Read the model definition and answer for the solid it produces. Units are mm, in the model's axes. Coordinates: 2 decimals unless noted, no trailing zeros. Order: outer loops, then holes, each group sorted by start corner. A loop starts at its lowest first (then second) coordinate and runs counter-clockwise, first axis right, second up. Notation, with made-up numbers: (58, 85) -> (110, 85) arc R4 ccw to (110, 90) -> close; hole circle Ø11 at (-10, -35). An arc over 180 degrees is marked (long way). Answer in a Markdown table with one row per item.
from build123d import *

# Parameters (mm, degrees)
SKETCH1_W           = 428.625
SKETCH1_H           = 47.625
BOSS_EXTRUDE1_DEPTH = 4.7625
SKETCH2_W           = 51.2445
SKETCH2_H           = 1.5875
SKETCH2_W_2         = 51.3715
CUT_EXTRUDE4_DEPTH  = 4.7625
SKETCH4_W           = 3.175
SKETCH4_H           = 44.45
CUT_EXTRUDE5_DEPTH  = 4.7625
SKETCH3_R           = 6.35
CUT_EXTRUDE6_DEPTH  = 4.7625


with BuildPart() as part:
    # Sketch1 → Boss-Extrude1 (new body)
    with BuildSketch(Plane(origin=(0, 0, 0), x_dir=(1, 0, 0), z_dir=(0, 1, 0))):
        Rectangle(SKETCH1_W, SKETCH1_H)
    extrude(amount=BOSS_EXTRUDE1_DEPTH)

    # Sketch2 → Cut-Extrude4 (cut)
    with BuildSketch(Plane.XZ):
        Polygon((-124.841, -22.225), (-124.841, -23.8125), (-19.05, -23.8125), (-19.05, -22.225), (-70.45325, -22.225), (-73.31075, -22.225), align=None)
        with Locations((188.69025, 23.01875)):
            Rectangle(SKETCH2_W, SKETCH2_H)
        Polygon((19.05, 23.8125), (19.05, 22.225), (70.58025, 22.225), (73.43775, 22.225), (124.968, 22.225), (124.968, 23.8125), align=None)
        Polygon((-124.841, 22.225), (-73.31075, 22.225), (-70.45325, 22.225), (-19.05, 22.225), (-19.05, 23.8125), (-124.841, 23.8125), align=None)
        Polygon((19.05, -22.225), (19.05, -23.8125), (124.968, -23.8125), (124.968, -22.225), (73.43775, -22.225), (70.58025, -22.225), align=None)
        with Locations((188.69025, -23.01875)):
            Rectangle(SKETCH2_W, SKETCH2_H)
        with Locations((-188.62675, 23.01875)):
            Rectangle(SKETCH2_W_2, SKETCH2_H)
        with Locations((-188.62675, -23.01875)):
            Rectangle(SKETCH2_W_2, SKETCH2_H)
        Polygon((-70.45325, -4.445), (-70.45325, -10.795), (-69.088, -10.795), (-69.088, -14.605), (-70.45325, -14.605), (-70.45325, -22.225), (-73.31075, -22.225), (-73.31075, -14.605), (-74.676, -14.605), (-74.676, -10.795), (-73.31075, -10.795), (-73.31075, -4.445), align=None)
        Polygon((-70.45325, 4.445), (-73.31075, 4.445), (-73.31075, 10.795), (-74.676, 10.795), (-74.676, 14.605), (-73.31075, 14.605), (-73.31075, 22.225), (-70.45325, 22.225), (-70.45325, 14.605), (-69.088, 14.605), (-69.088, 10.795), (-70.45325, 10.795), align=None)
        Polygon((73.43775, 4.445), (70.58025, 4.445), (70.58025, 10.795), (69.215, 10.795), (69.215, 14.605), (70.58025, 14.605), (70.58025, 22.225), (73.43775, 22.225), (73.43775, 14.605), (74.803, 14.605), (74.803, 10.795), (73.43775, 10.795), align=None)
        Polygon((73.43775, -4.445), (73.43775, -10.795), (74.803, -10.795), (74.803, -14.605), (73.43775, -14.605), (73.43775, -22.225), (70.58025, -22.225), (70.58025, -14.605), (69.215, -14.605), (69.215, -10.795), (70.58025, -10.795), (70.58025, -4.445), align=None)
    extrude(amount=-CUT_EXTRUDE4_DEPTH, mode=Mode.SUBTRACT)

    # Sketch4 → Cut-Extrude5 (cut)
    with BuildSketch(Plane.XZ):
        with Locations((-212.725, 0)):
            Rectangle(SKETCH4_W, SKETCH4_H)
        with Locations((212.725, 0)):
            Rectangle(SKETCH4_W, SKETCH4_H)
    extrude(amount=-CUT_EXTRUDE5_DEPTH, mode=Mode.SUBTRACT)

    # Sketch3 → Cut-Extrude6 (cut)
    with BuildSketch(Plane.XZ):
        with Locations(Location((-143.891, 0, 0), (0, 0, 270))):
            Circle(SKETCH3_R)
        with Locations(Location((144.018, 0, 0), (0, 0, 270))):
            Circle(SKETCH3_R)
    extrude(amount=-CUT_EXTRUDE6_DEPTH, mode=Mode.SUBTRACT)


solid = part.part
Q1. The part is cut by section A-A (z = 0). Write down the section's boundary in (x, y), then the cut area to 3 significant figures.
Outcome:
| item | result |
|---|---|
| outline | (-211.14, 0) -> (-150.24, 0) -> (-150.24, 4.76) -> (-211.14, 4.76) -> close; (-137.54, 0) -> (137.67, 0) -> (137.67, 4.76) -> (-137.54, 4.76) -> close; (150.37, 0) -> (211.14, 0) -> (211.14, 4.76) -> (150.37, 4.76) -> close |
| area | 1,890 mm² |
Q2. The part is cut by section C-C (y = 2.45). Give the number of separate pieces and of enclosed holes in the cut face, then the cut area to 3 significant figures.
Outcome:
| item | result |
|---|---|
| separate pieces | 1 |
| enclosed holes | 2 |
| area | 18,600 mm² |
Q3. Consider line 1 (X direction, y = 2.5, z = -8); line 2 (X direction, y = 1.4, z = 11) (1 decimal); line 3 (X direction, y = 4.05, z = 5). Determine where each line is inside the solid, lowest interval first.
Outcome:
| item | result |
|---|---|
| line 1 | -211.14 to -73.31, -70.45 to 70.58, 73.44 to 211.14 |
| line 2 | -211.1 to -74.7, -69.1 to 69.2, 74.8 to 211.1 |
| line 3 | -211.14 to -147.81, -139.98 to -73.31, -70.45 to 70.58, 73.44 to 140.1, 147.93 to 211.14 |
Q4. The part is cut by section B-B (x = 84). Write down the section's boundary in (y, z) (1 decimal), then the cut area to 3 significant figures.
Outcome:
| item | result |
|---|---|
| outline | (0, -22.2) -> (4.8, -22.2) -> (4.8, 22.2) -> (0, 22.2) -> close |
| area | 212 mm² |
Q5. Given pin 1 (1.3 mm diameter, centred on y = 3.5, z = 23.5, fed in from +X); pin 2 (1.3 mm diameter, centred on y = 1, z = -23, fed in from -X); pin 3 (2.5 mm diameter, centred on x = -106, y = 1, fed in from +Z) (3 decimals), each flat-ended and moving along its own axis, determine where each tip first touches the part or whether it passes through.
Outcome:
| item | result |
|---|---|
| pin 1 | x = 163.07 |
| pin 2 | x = -162.94 |
| pin 3 | z = 22.225 |
Q6. For a pull along X with two mould halves and no side action, classify faces 1 (the face through (150.314, 2.348, 0.827)), 2 (the face through (-3, 4.762, 0)) as pulls with the +X half, pulls with the -X half, needs draft (parallel to the pull), parting line crosses it, or undercut.
Outcome:
| item | result |
|---|---|
| face 1 | undercut |
| face 2 | needs draft |
